from build123d import *

# Parameters (mm, degrees)
BOSS_EXTRUDE1_DEPTH = 7
CUT_EXTRUDE1_DEPTH  = 28.51
SKETCH4_R           = 1.6
CUT_EXTRUDE2_DEPTH  = 3
SKETCH5_R           = 1.6
CUT_EXTRUDE3_DEPTH  = 3
SKETCH6_W           = 7
SKETCH6_H           = 0.3
CUT_EXTRUDE4_DEPTH  = 28.51
SKETCH8_W           = 7
SKETCH8_H           = 1.7
CUT_EXTRUDE6_DEPTH  = 1
SKETCH9_W           = 2.5
SKETCH9_H           = 7
BOSS_EXTRUDE2_DEPTH = 3
CUT_EXTRUDE7_DEPTH  = 7
CHAMFER1_SIZE       = 1
SKETCH11_W          = 7
SKETCH11_H          = 1.7
CUT_EXTRUDE8_DEPTH  = 1


with BuildPart() as part:
    # Sketch1 → Boss-Extrude1 (new body)
    with BuildSketch(Plane.XY):
        Polygon((17.01, -5), (17.01, -3), (8.51, -3), (8.51, -5), (8.41, -5), (-2.8, -5), (-2.9, -5), (-2.9, -3), (-11.5, -3), (-11.5, -5), (-11.6, -5), (-16.6, -5), (-16.6, -8), (22.11, -8), (22.11, -5), (17.11, -5), align=None)
    extrude(amount=-BOSS_EXTRUDE1_DEPTH)

    # Sketch2 → Cut-Extrude1 (cut)
    with BuildSketch(Plane.ZY.offset(11.5)):
        Polygon((0, -3), (-1, -3), (-1, -4), (-2, -4), (-2, -3), (-3, -3), (-3, -4), (-4, -4), (-4, -3), (-5, -3), (-5, -4), (-6, -4), (-6, -3), (-7, -3), (-7, -2.645827001), (0, -2.645827001), align=None)
    extrude(amount=-CUT_EXTRUDE1_DEPTH, mode=Mode.SUBTRACT)

    # Sketch4 → Cut-Extrude2 (cut)
    with BuildSketch(Plane(origin=(0, -5, 0), x_dir=(1, 0, 0), z_dir=(0, 1, 0))):
        with Locations((2.805, 3.5)):
            Circle(SKETCH4_R)
    extrude(amount=-CUT_EXTRUDE2_DEPTH, mode=Mode.SUBTRACT)

    # Sketch5 → Cut-Extrude3 (cut)
    with BuildSketch(Plane(origin=(0, -5, 0), x_dir=(1, 0, 0), z_dir=(0, 1, 0))):
        with Locations((-14.05, 3.5)):
            Circle(SKETCH5_R)
        with Locations((19.56, 3.5)):
            Circle(SKETCH5_R)
    extrude(amount=-CUT_EXTRUDE3_DEPTH, mode=Mode.SUBTRACT)

    # Sketch6 → Cut-Extrude4 (cut)
    with BuildSketch(Plane(origin=(17.01, 0, 0), x_dir=(0, 0, -1), z_dir=(1, 0, 0))):
        with Locations((3.5, -3.15)):
            Rectangle(SKETCH6_W, SKETCH6_H)
    extrude(amount=-CUT_EXTRUDE4_DEPTH, mode=Mode.SUBTRACT)

    # Sketch8 → Cut-Extrude6 (cut)
    with BuildSketch(Plane.ZY.offset(11.5)):
        with Locations((-3.5, -4.15)):
            Rectangle(SKETCH8_W, SKETCH8_H)
    extrude(amount=-CUT_EXTRUDE6_DEPTH, mode=Mode.SUBTRACT)

    # Sketch9 → Boss-Extrude2 (add)
    with BuildSketch(Plane.XZ.offset(8)):
        with Locations((-17.85, -3.5)):
            Rectangle(SKETCH9_W, SKETCH9_H)
        with Locations((23.36, -3.5)):
            Rectangle(SKETCH9_W, SKETCH9_H)
    extrude(amount=-BOSS_EXTRUDE2_DEPTH)

    # Sketch10 → Cut-Extrude7 (cut)
    with BuildSketch(Plane(origin=(0, 0, -7), x_dir=(-1, 0, 0), z_dir=(0, 0, -1))):
        with BuildLine():
            Line((-17.01, -8), (-8.51, -8))
            ThreePointArc((-8.51, -8), (-12.76, -6.3), (-17.01, -8))
        make_face()
        with BuildLine():
            Line((2.9, -8), (10.5, -8))
            ThreePointArc((10.5, -8), (6.7, -6.601279457), (2.9, -8))
        make_face()
    extrude(amount=-CUT_EXTRUDE7_DEPTH, mode=Mode.SUBTRACT)

    # Chamfer1
    chamfer1_edges = [part.edges().sort_by_distance(p)[0] for p in [
        (-19.1, -6.5, -7),
        (-19.1, -6.5, 0),
        (24.61, -6.5, 0),
        (24.61, -6.5, -7),
    ]]
    chamfer(chamfer1_edges, length=CHAMFER1_SIZE)

    # Sketch11 → Cut-Extrude8 (cut)
    with BuildSketch(Plane(origin=(17.01, 0, 0), x_dir=(0, 0, -1), z_dir=(1, 0, 0))):
        with Locations((3.5, -4.15)):
            Rectangle(SKETCH11_W, SKETCH11_H)
    extrude(amount=-CUT_EXTRUDE8_DEPTH, mode=Mode.SUBTRACT)


solid = part.part
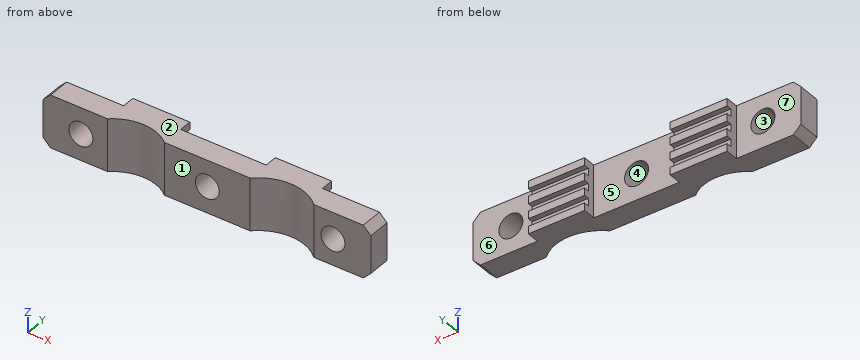
CAD build for the part. Positions are in the model's coordinates, mm. Face numbers are marked on the shaded views. A direction names the side the tool comes from. Round coordinates to 2 decimals unless told otherwise and drop trailing zeros. Loops run counter-clockwise (first coordinate to the right, second up) from the corner with the lowest first, then second, coordinate; pieces in that order, holes last.
(1) Cut at C-C (y = -5.4). Give the cut face in (x, z) (3 decimals).
(2) Cut at A-A (x = 19.56). Give the cut face in (y, z).
(3) Cut at D-D (z = -0.5). Give the cut face in (x, y) (1 decimal), plus the area to 3 significant figures.
(4) Two-plate mould, pull along Z, no slides. Class the marked faces 1, 2, 3 and 4: +Z half, -Z half, draft (parallel to the pull), parting line (faces both ways), or undercut.
(5) Wall check: line 1 along X through (y, z) = (-6.05, -3.5) (3 decimals); line 2 along Z through (x, y) = (19.56, -5.7); line 3 along X through (y, z) = (-7.7, -3). Give the ranges that are in metal, low to high.
(6) Drop flat-ended pins along their axis: pin 1 (0.8 mm diameter, centred on y = -4, z = -3, fed in from +X); pin 2 (4 mm diameter, centred on x = -7, z = -2, fed in from -Y); pin 3 (0.8 mm diameter, centred on x = 11.5, z = -5.5, fed in from +Y). Give the stop position or say it passes through.
(7) Cut at B-B (z = -3.5). State how many separate pieces and enclosed holes the cut face has, plus the area to 3 significant figures.
(8) Which spindle directions (+Z, -Z, +X, -X, +Y, -Y) get a long thin tool onto all of the face, cutting with end or side? Do the marked faces 5, 6 and 7. Say none if no direction does.
Findings below:
1. outline: (-19.1, -6) - (-18.1, -7) - (23.61, -7) - (24.61, -6) - (24.61, -1) - (23.61, 0) - (-18.1, 0) - (-19.1, -1) - close; hole circle Ø3.2 at (-14.05, -3.5); hole circle Ø3.2 at (2.805, -3.5); hole circle Ø3.2 at (19.56, -3.5)
2. outline: (-8, -7) - (-5, -7) - (-5, -5.1) - (-8, -5.1) - close; (-8, -1.9) - (-5, -1.9) - (-5, 0) - (-8, 0) - close
3. outline: (-18.6, -8) - (-10.5, -8) arc R5.9 cw to (-2.9, -8) - (8.5, -8) arc R6.2 cw to (17, -8) - (24.1, -8) - (24.1, -5) - (16, -5) - (16, -3.3) - (8.5, -3.3) - (8.5, -5) - (-2.9, -5) - (-2.9, -3.3) - (-10.5, -3.3) - (-10.5, -5) - (-18.6, -5) - close
3. area: 137 mm2
4. face 1: draft
4. face 2: +Z half
4. face 3: undercut
4. face 4: undercut
5. line 1: x = -19.1 to -15.65, -12.45 to 1.205, 4.405 to 17.96, 21.16 to 24.61
5. line 2: z = -7 to -5.1, -1.9 to 0
5. line 3: x = -19.1 to -15.57, -12.53 to -10.12, -3.28 to 1.29, 4.32 to 8.85, 16.67 to 18.04, 21.08 to 24.61
6. pin 1: stops at x = 16.01
6. pin 2: stops at y = -7.07
6. pin 3: stops at y = -4
7. separate pieces: 4
7. enclosed holes: 0
7. area: 100 mm2
8. face 5: +Z, -Z, +Y
8. face 6: +Z, -Z, +X, +Y
8. face 7: +Z, -Z, -X, +Y
